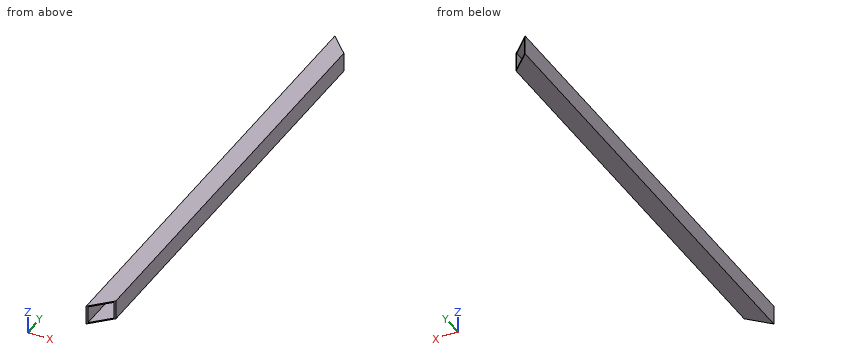
```python
from build123d import *

# Parameters (mm, degrees)
F0_W     = 38.1
F0_H     = 38.1
F0_W_2   = 33.528
F0_H_2   = 33.528
F1_DEPTH = 914.4
F3_DEPTH = 50.8


with BuildPart() as f1:
    # F0 (on Front) → F1 (new body)
    with BuildSketch(Plane.XZ):
        with Locations((-19.05, -19.05)):
            Rectangle(F0_W, F0_H)
        with Locations((-19.05, -19.05)):
            Rectangle(F0_W_2, F0_H_2, mode=Mode.SUBTRACT)
    extrude(amount=F1_DEPTH)

    # F2 (on face) → F3 (cut)
    with BuildSketch(Plane.XY):
        Polygon((0, -876.3), (-38.1, -914.4), (0, -914.4), align=None)
        Polygon((0, 0), (-38.1, 0), (0, -38.1), align=None)
    extrude(amount=-F3_DEPTH, mode=Mode.SUBTRACT)


solid = f1.part
```
Here's how the part is built. I have some questions about the finished solid (model axes, mm). Round coordinates to 2 decimals unless told otherwise and drop trailing zeros. Order: outer loops, then holes, each group sorted by start corner. A loop starts at its lowest first (then second) coordinate and runs counter-clockwise, first axis right, second up. Notation, with made-up numbers: (73, -12) -> (85, -12) arc R10 cw to (85, 0) -> close; hole circle Ø5 at (19, 5.5). An arc over 180 degrees is marked (long way). Use a Markdown table: item, result. Add a question column.
(1) I need wall thicknesses on line 1 along Z through (x, y) = (-18.5, -455). Which ranges of the line are inside material? Lowest first, please.
(2) Suppose I cut it at A-A, the plane x = -19. Please give me the cut outline in (y, z), and give its area (3 significant figures).
(3) Suppose I cut it at B-B, the plane z = -20.5. Please give me the cut outline in (x, y).
(4) Suppose I cut it at C-C, the plane y = -204. Please give me the cut outline in (x, z).
(5) For pin 1 Ø3 at (y, z) = (-743, -9) entering from +X, with a flat end and sliding along its axis, tell me the tip position at first contact or that it passes through.
Verdict:
| question | item | result |
|---|---|---|
| 1 | line 1 | -38.1 to -35.81, -2.29 to 0 |
| 2 | outline | (-895.3, -38.1) -> (-19.1, -38.1) -> (-19.1, -35.81) -> (-895.3, -35.81) -> close; (-895.3, -2.29) -> (-19.1, -2.29) -> (-19.1, 0) -> (-895.3, 0) -> close |
| 2 | area | 4,010 mm2 |
| 3 | outline | (-38.1, -914.4) -> (-35.81, -912.11) -> (-35.81, -2.29) -> (-38.1, 0) -> close; (-2.29, -878.59) -> (0, -876.3) -> (0, -38.1) -> (-2.29, -35.81) -> close |
| 4 | outline | (-38.1, -38.1) -> (0, -38.1) -> (0, 0) -> (-38.1, 0) -> close; hole (-35.81, -35.81) -> (-2.29, -35.81) -> (-2.29, -2.29) -> (-35.81, -2.29) -> close |
| 5 | pin 1 | x = 0 |
